```python
from build123d import *

# Parameters (mm, degrees)
CYLINDER119_R           = 1.5
CYLINDER119_DEPTH       = 8
CYLINDER121_R           = 2.5
CYLINDER121_DEPTH       = 8
CYLINDER122_R           = 2.5
CYLINDER122_DEPTH       = 8
CYLINDER123_R           = 2.5
CYLINDER123_DEPTH       = 8
CYLINDER124_R           = 2.5
CYLINDER124_DEPTH       = 8
CYLINDER126_R           = 2.1
CYLINDER126_DEPTH       = 5
CYLINDER118_R           = 1.5
CYLINDER118_DEPTH       = 8
CYLINDER128_R           = 0.4
CYLINDER128_DEPTH       = 9
CYLINDER128_PITCH_ANGLE = 90
BOX023_W                = 3
BOX023_H                = 6
BOX023_DEPTH            = 4.5
CYLINDER127_R           = 1.5
CYLINDER127_DEPTH       = 8
CYLINDER120_R           = 1.5
CYLINDER120_DEPTH       = 8
BOX021_W                = 20
BOX021_H                = 6
BOX021_DEPTH            = 4.5
CYLINDER129_R           = 0.4
CYLINDER129_DEPTH       = 10
CYLINDER130_R           = 2.1
CYLINDER130_DEPTH       = 2


with BuildPart() as bowtiemount1:
    # Cylinder119 → Cylinder119 (new body)
    with BuildSketch(Plane(origin=(114, 151, 63), x_dir=(1, 0, 0), z_dir=(0, 0, 1))):
        Circle(CYLINDER119_R)
    extrude(amount=CYLINDER119_DEPTH)


with BuildPart() as bowtiecut1:
    # Cylinder121 → Cylinder121 (new body)
    with BuildSketch(Plane(origin=(125.5, 145, 64), x_dir=(1, 0, 0), z_dir=(0, 0, 1))):
        Circle(CYLINDER121_R)
    extrude(amount=CYLINDER121_DEPTH)


with BuildPart() as bowtiecut2:
    # Cylinder122 → Cylinder122 (new body)
    with BuildSketch(Plane(origin=(125.5, 152, 64), x_dir=(1, 0, 0), z_dir=(0, 0, 1))):
        Circle(CYLINDER122_R)
    extrude(amount=CYLINDER122_DEPTH)


with BuildPart() as bowtiecut3:
    # Cylinder123 → Cylinder123 (new body)
    with BuildSketch(Plane(origin=(118.5, 152, 64), x_dir=(1, 0, 0), z_dir=(0, 0, 1))):
        Circle(CYLINDER123_R)
    extrude(amount=CYLINDER123_DEPTH)


with BuildPart() as bowtiecut4:
    # Cylinder124 → Cylinder124 (new body)
    with BuildSketch(Plane(origin=(118.5, 144.5, 64), x_dir=(1, 0, 0), z_dir=(0, 0, 1))):
        Circle(CYLINDER124_R)
    extrude(amount=CYLINDER124_DEPTH)


with BuildPart() as bowtienozzlecut:
    # Cylinder126 → Cylinder126 (new body)
    with BuildSketch(Plane(origin=(122, 148.5, 68.5), x_dir=(1, 0, 0), z_dir=(0, 0, 1))):
        Circle(CYLINDER126_R)
    extrude(amount=CYLINDER126_DEPTH)


with BuildPart() as bowtiecruciblehole:
    # Cylinder118 → Cylinder118 (new body)
    with BuildSketch(Plane(origin=(122, 148.5, 66), x_dir=(1, 0, 0), z_dir=(0, 0, 1))):
        Circle(CYLINDER118_R)
    extrude(amount=CYLINDER118_DEPTH)


with BuildPart() as bowtieinjector:
    # Cylinder128 → Cylinder128 (new body)
    with BuildSketch(Plane.XY):
        Circle(CYLINDER128_R)
    extrude(amount=CYLINDER128_DEPTH)


with BuildPart() as bowtieinjector_1:
    # Cylinder128 pitch: moved
    add(bowtieinjector.part.rotate(Axis((0, 0, 0), (0, 1, 0)), CYLINDER128_PITCH_ANGLE))


with BuildPart() as bowtieinjector_2:
    # Cylinder128 placement: moved
    add(bowtieinjector_1.part.moved(Location((112, 148.5, 68))))


with BuildPart() as bowtiecut5:
    # Box023 → Box023 (new body)
    with BuildSketch(Plane(origin=(125, 145.5, 73), x_dir=(1, 0, 0), z_dir=(0, 0, 1))):
        with Locations((1.5, 3)):
            Rectangle(BOX023_W, BOX023_H)
    extrude(amount=BOX023_DEPTH)


with BuildPart() as bowtiemount007:
    # Cylinder127 → Cylinder127 (new body)
    with BuildSketch(Plane(origin=(114, 146, 63), x_dir=(1, 0, 0), z_dir=(0, 0, 1))):
        Circle(CYLINDER127_R)
    extrude(amount=CYLINDER127_DEPTH)


with BuildPart() as fusion050:
    # Cylinder120 → Cylinder120 (new body)
    with BuildSketch(Plane(origin=(130, 148.5, 63), x_dir=(1, 0, 0), z_dir=(0, 0, 1))):
        Circle(CYLINDER120_R)
    extrude(amount=CYLINDER120_DEPTH)

    # Fusion050: union BowTieMount1, BowTieCut1, BowTieCut2, BowTieCut3, BowTieCut4, BowTieNozzleCut, BowTieCrucibleHole, BowTieInjector, BowTieCut5, BowTieMount007
    add(bowtiemount1.part)
    add(bowtiecut1.part)
    add(bowtiecut2.part)
    add(bowtiecut3.part)
    add(bowtiecut4.part)
    add(bowtienozzlecut.part)
    add(bowtiecruciblehole.part)
    add(bowtieinjector_2.part)
    add(bowtiecut5.part)
    add(bowtiemount007.part)


with BuildPart() as bowtie:
    # Box021 → Box021 (new body)
    with BuildSketch(Plane(origin=(112, 145.5, 65), x_dir=(1, 0, 0), z_dir=(0, 0, 1))):
        with Locations((10, 3)):
            Rectangle(BOX021_W, BOX021_H)
    extrude(amount=BOX021_DEPTH)

    # Cut015: cut Fusion050
    add(fusion050.part, mode=Mode.SUBTRACT)


with BuildPart() as bowtie_1:
    # Cut015 placement: moved
    add(bowtie.part.moved(Location((-16.5, 0, 0))))


with BuildPart() as bowtienozzle001:
    # Cylinder129 → Cylinder129 (new body)
    with BuildSketch(Plane(origin=(122, 148.5, 68), x_dir=(1, 0, 0), z_dir=(0, 0, 1))):
        Circle(CYLINDER129_R)
    extrude(amount=CYLINDER129_DEPTH)


with BuildPart() as cone:
    # Cone → Cone (revolve)
    with BuildSketch(Plane(origin=(122, 148.5, 70), x_dir=(1, 0, 0), z_dir=(0, -1, 0))):
        Polygon((0, 0), (2.1, 0), (1, 5), (0, 5), align=None)
    revolve(axis=Axis((122, 148.5, 70), (0, 0, 1)))


with BuildPart() as fusion055:
    # Cylinder130 → Cylinder130 (new body)
    with BuildSketch(Plane(origin=(122, 148.5, 68), x_dir=(1, 0, 0), z_dir=(0, 0, 1))):
        Circle(CYLINDER130_R)
    extrude(amount=CYLINDER130_DEPTH)

    # Fusion051: union Cone
    add(cone.part)

    # Cut016: cut BowTieNozzle001
    add(bowtienozzle001.part, mode=Mode.SUBTRACT)


with BuildPart() as fusion055_1:
    # Cut016 placement: moved
    add(fusion055.part.moved(Location((-16.5, 0, 0))))

    # Fusion055: union BowTie
    add(bowtie_1.part)


solid = fusion055_1.part
```
The listing builds one solid part. Answer for the finished solid, in the listing's coordinates (mm). A direction names the side the tool comes from. Coordinates: 2 decimals unless noted, no trailing zeros. Write each loop counter-clockwise with the first axis right and the second up, starting at its lowest first coordinate (ties: lowest second). Pieces come first, ordered by that corner, then holes. Notation, with made-up numbers: M 83.25,51.5 L 142.25,51.5 A18 ccw 142.25,64.5 Z; hole C -27.5,24.25 d3. An arc over 180 degrees is marked long. Use a Markdown table: item, result. Add a question column.
1. Section C-C (z = 67) is taken. Give the vertices of the cut face in (x, y).
2. Section B-B (x = 113.5) is taken. Give the vertices of the cut face in (y, z), plus the area to 3 significant figures.
3. Which of the six approach directions +Z, -Z, +X, -X, +Y, -Y give full straight-line access (tool end or side, diameter ignored) to faces 5 (the flat face through (105, 149, 66)), 6 (the flat face through (105, 149, 65)), 7 (the cylindrical face through (99.72, 148.35, 67.63))?
4. Straight lines are drawn through the part: line 1 along Y through (x, z) = (113.5, 66.15); line 2 along Z through (x, y) = (101.5, 148.5); line 3 along X through (y, z) = (148.2, 66.5). For each, find the intervals that lie inside material, in ascending order. Write a range as [from, to].
5. For a pull along Y with two mould halves and no side action, classify faces 1 (the cylindrical face through (112.39, 149.51, 67.22)), 2 (the cylindrical face through (103.952, 149.919, 69.746)), 3 (the flat face through (115.5, 148, 67)), 4 (the flat face through (113, 145.5, 67)) as +Y half, -Y half, draft (parallel to the pull), parting line (faces both ways), or undercut.
6. Section D-D (y = 151) is taken. Give the vertices of the cut face in (x, z), plus the area to 3 significant figures.
7. Section A-A (y = 148.5) is taken. Give the vertices of the cut face in (x, z).
8. Given P1, Ø2, axis at x = 107, y = 147.5, coming from the +Z side; P2, Ø1, axis at x = 99.5, y = 151, coming from the +Z side, each flat-ended and moving along its own axis, determine where each tip first touches the part or whether it passes through.
Data:
| question | item | result |
|---|---|---|
| 1 | outline | M 95.5,145.5 L 96.09,145.5 A1.5 cw long 98.91,145.5 L 99.71,145.5 A2.5 cw 104.29,145.5 L 106.55,145.5 A2.5 cw 111.45,145.5 L 115.5,145.5 L 115.5,151.5 L 111.45,151.5 A2.5 cw 106.55,151.5 L 104.45,151.5 A2.5 cw 99.55,151.5 L 98.91,151.5 A1.5 cw long 96.09,151.5 L 95.5,151.5 Z; hole C 105.5,148.5 d3; hole C 113.5,148.5 d3 |
| 2 | outline | M 145.5,65 L 147,65 L 147,69.5 L 145.5,69.5 Z; M 150,65 L 151.5,65 L 151.5,69.5 L 150,69.5 Z |
| 2 | area | 13.5 mm2 |
| 3 | face 5 | none |
| 3 | face 6 | -Z, +X, -X, +Y, -Y |
| 3 | face 7 | -X |
| 4 | line 1 | y = [145.5, 147], [150, 151.5] |
| 4 | line 2 | z = [65, 67.6], [68.4, 69.5] |
| 4 | line 3 | x = [95.5, 104.03], [106.97, 112.03], [114.97, 115.5] |
| 5 | face 1 | undercut |
| 5 | face 2 | parting line |
| 5 | face 3 | draft |
| 5 | face 4 | -Y half |
| 6 | outline | M 95.5,65 L 96,65 L 96,69.5 L 95.5,69.5 Z; M 99,65 L 99.71,65 L 99.71,69.5 L 99,69.5 Z; M 104.29,65 L 106.71,65 L 106.71,69.5 L 104.29,69.5 Z; M 111.29,65 L 115.5,65 L 115.5,69.5 L 111.29,69.5 Z |
| 6 | area | 35.3 mm2 |
| 7 | outline | M 95.5,65 L 112,65 L 112,69.5 L 107.6,69.5 L 107.6,70 L 106.5,75 L 105.9,75 L 105.9,68 L 107,68 L 107,66 L 104,66 L 104,67.6 L 95.5,67.6 Z; M 95.5,68.4 L 103.4,68.4 L 103.4,68 L 105.1,68 L 105.1,75 L 104.5,75 L 103.4,70 L 103.4,69.5 L 95.5,69.5 Z; M 115,65 L 115.5,65 L 115.5,69.5 L 115,69.5 Z |
| 8 | P1 | stops at z = 75 |
| 8 | P2 | stops at z = 69.5 |
